Geometry: see drawing. Coordinates: mm, zero at the bounding-box minimum. Give positions to 0.01 mm unless a question says otherwise; leave off trailing zeros. Loops run counter-clockwise (first coordinate to the right, second up) from the corner with the lowest first, then second, coordinate; pieces in that order, holes last. Notation, with made-up numbers: (53.5, 5) - (60.5, 5) arc R13 ccw to (60.5, 26) - close; hole circle Ø7 at (8, -35.75). An arc over 180 degrees is marked (long way). Use CSV: the item, a comma, the result in double quotes. Start each with the question number.
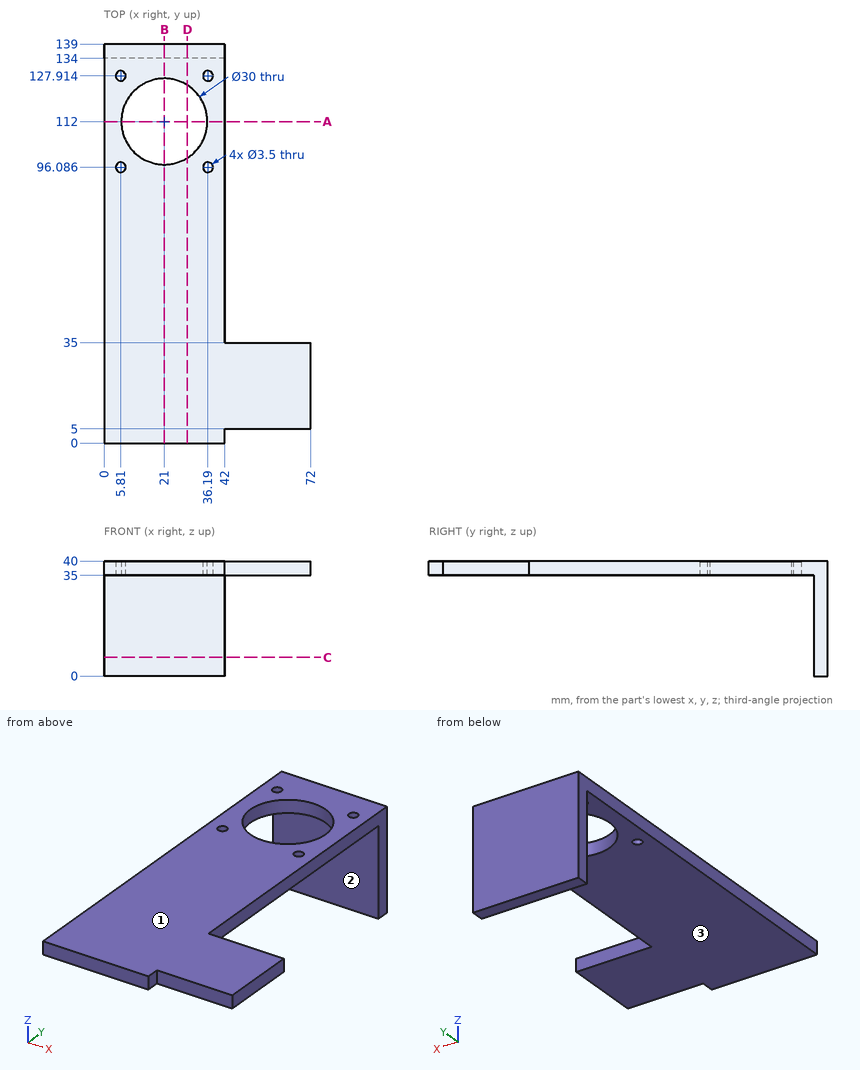
Item 1: Ray query, probe 1 along Y at (x, z) = (21, 37.8); probe 2 along Y at (x, z) = (33.5, 26); probe 3 along X at (y, z) = (50.5, 35.5). Return the intervals inside material, ascending.
Item 2: Section B-B (x = 21). Output: boundary loops of the cut face in (y, z).
Item 3: Section C-C (z = 6.5). Output: boundary loops of the cut face in (x, y).
Item 4: Section D-D (x = 29). Output: boundary loops of the cut face in (y, z).
Item 5: Pin query (flat end, axial travel): pin 1 Ø12 at (x, y) = (20, 91) entering from -Z; pin 2 Ø2.5 at (x, z) = (62.5, 36.5) entering from +Y; pin 3 Ø5 at (x, z) = (33, 20.5) entering from -Y; pin 4 Ø5.5 at (y, z) = (3.5, 36.5) entering from +X. Return the tip coordinate at first contact, or that it passes through.
Item 6: Section A-A (y = 112). Output: boundary loops of the cut face in (x, z), plus the area to 3 significant figures.
Item 7: Mould query, pull axis Z, two halves, no side actions, for the marked faces 1, 2 and 3. Classes: pulls with the +Z half, pulls with the -Z half, needs draft (parallel to the pull), parting line crosses it, or undercut.
Outcome:
1,probe 1,"y = 0 to 97, 127 to 139"
1,probe 2,"y = 134 to 139"
1,probe 3,"x = 0 to 42"
2,outline,"(0, 35) - (97, 35) - (97, 40) - (0, 40) - close; (127, 35) - (134, 35) - (134, 0) - (139, 0) - (139, 40) - (127, 40) - close"
3,outline,"(0, 134) - (42, 134) - (42, 139) - (0, 139) - close"
4,outline,"(0, 35) - (99.31, 35) - (99.31, 40) - (0, 40) - close; (124.69, 35) - (134, 35) - (134, 0) - (139, 0) - (139, 40) - (124.69, 40) - close"
5,pin 1,"stops at z = 35"
5,pin 2,"stops at y = 35"
5,pin 3,"stops at y = 134"
5,pin 4,"stops at x = 72"
6,outline,"(0, 35) - (6, 35) - (6, 40) - (0, 40) - close; (36, 35) - (42, 35) - (42, 40) - (36, 40) - close"
6,area,"60.0 mm2"
7,face 1,"pulls with the +Z half"
7,face 2,"needs draft"
7,face 3,"pulls with the -Z half"
